For this review, take the finished solid that the model builds, in its own axes (mm). Face numbers are marked on the shaded views. Coordinates: 2 decimals unless noted, no trailing zeros. Loops run counter-clockwise (first coordinate to the right, second up) from the corner with the lowest first, then second, coordinate; pieces in that order, holes last. Notation, with made-up numbers: (66.5, 74) -> (88.5, 74) arc R31 ccw to (88.5, 105) -> close; hole circle Ø2 at (5.5, -3.75). An arc over 180 degrees is marked (long way). Use a Markdown table: item, result.
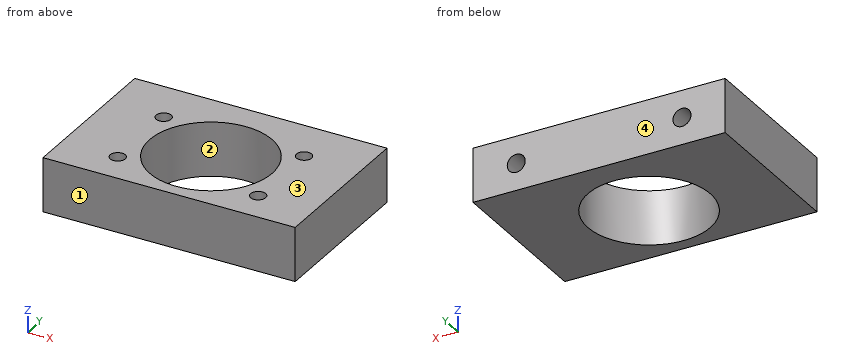
from build123d import *

# Parameters (mm, degrees)
SKETCH_1_W             = 70
SKETCH_1_H             = 45
EXTRUDE_1_DEPTH        = 15
SKETCH_2_R             = 17
CUT_EXTRUDE_1_DEPTH    = 85.557672626
HOLE_WIZARD_M6_1_D     = 5
HOLE_WIZARD_M6_1_DEPTH = 15
HOLE_WIZARD_M6_1_TIP   = 1.502151548
HOLE_WIZARD_M5_1_D     = 4.2
HOLE_WIZARD_M5_1_DEPTH = 12.4
HOLE_WIZARD_M5_1_TIP   = 1.2618073


with BuildPart() as part:
    # 草图1 → 凸台-拉伸1 (new body)
    with BuildSketch(Plane.XY):
        with Locations((35, 22.5)):
            Rectangle(SKETCH_1_W, SKETCH_1_H)
    extrude(amount=EXTRUDE_1_DEPTH)

    # 草图2 → 切除-拉伸1 (cut, through all)
    with BuildSketch(Plane.XY.offset(15)):
        with Locations((35, 20.5)):
            Circle(SKETCH_2_R)
    extrude(amount=-CUT_EXTRUDE_1_DEPTH, mode=Mode.SUBTRACT)

    # M6 螺纹孔1
    with Locations(Plane(origin=(0, 45, 0), x_dir=(-1, 0, 0), z_dir=(0, 1, 0))):
        with Locations((-12, 7.5), (-58, 7.5)):
            Hole(HOLE_WIZARD_M6_1_D / 2, depth=HOLE_WIZARD_M6_1_DEPTH)
            with Locations((0, 0, -(HOLE_WIZARD_M6_1_DEPTH + HOLE_WIZARD_M6_1_TIP / 2))):  # 118° drill point
                Cone(0, HOLE_WIZARD_M6_1_D / 2, HOLE_WIZARD_M6_1_TIP, mode=Mode.SUBTRACT)

    # M5 螺纹孔1
    with Locations(Plane.XY.offset(15)):
        with Locations((54.485571585, 31.75), (15.514428415, 31.75), (54.485571585, 9.25), (15.514428415, 9.25)):
            Hole(HOLE_WIZARD_M5_1_D / 2, depth=HOLE_WIZARD_M5_1_DEPTH)
            with Locations((0, 0, -(HOLE_WIZARD_M5_1_DEPTH + HOLE_WIZARD_M5_1_TIP / 2))):  # 118° drill point
                Cone(0, HOLE_WIZARD_M5_1_D / 2, HOLE_WIZARD_M5_1_TIP, mode=Mode.SUBTRACT)


solid = part.part
(1) Take a section at C-C on z = 11. Write out the cut boundary in (x, y).
Found:
| item | result |
|---|---|
| outline | (0, 0) -> (70, 0) -> (70, 45) -> (0, 45) -> close; hole circle Ø4.2 at (15.51, 9.25); hole circle Ø4.2 at (15.51, 31.75); hole circle Ø34 at (35, 20.5); hole circle Ø4.2 at (54.49, 9.25); hole circle Ø4.2 at (54.49, 31.75) |
(2) Take a section at D-D on y = 27. Write out the cut boundary in (x, z), plus the area to 3 significant figures.
Found:
| item | result |
|---|---|
| outline | (0, 0) -> (19.29, 0) -> (19.29, 15) -> (0, 15) -> close; (50.71, 0) -> (70, 0) -> (70, 15) -> (50.71, 15) -> close |
| area | 579 mm^2 |
(3) For line 1 along Y through (x, z) = (54.5, 4.25); line 2 along X through (y, z) = (32, 2.5); line 3 along Y through (x, z) = (35, 8), list the stretches that pass through material, from the lowest coordinate up.
Found:
| item | result |
|---|---|
| line 1 | y = 0 to 7.15, 11.35 to 29.65, 33.85 to 45 |
| line 2 | x = 0 to 13.6, 17.43 to 22.48, 47.52 to 52.57, 56.4 to 70 |
| line 3 | y = 0 to 3.5, 37.5 to 45 |
(4) Mouldability with a two-part tool opening along Y and no side actions: class the marked faces 1, 2, 3 and 4 as pulls with the +Y half, pulls with the -Y half, needs draft (parallel to the pull), parting line crosses it, or undercut.
Found:
| item | result |
|---|---|
| face 1 | pulls with the -Y half |
| face 2 | undercut |
| face 3 | needs draft |
| face 4 | pulls with the +Y half |
(5) Take a section at B-B on y = 36.5. Write out the cut boundary in (x, z), plus the area to 3 significant figures.
Found:
| item | result |
|---|---|
| outline | (0, 0) -> (29.26, 0) -> (29.26, 15) -> (0, 15) -> close; (40.74, 0) -> (70, 0) -> (70, 15) -> (40.74, 15) -> close; hole circle Ø5 at (12, 7.5); hole circle Ø5 at (58, 7.5) |
| area | 838 mm^2 |
(6) For pin 1 Ø3.5 at (x, y) = (54.49, 31.75) entering from +Z, flat-tipped, find the tip position at first contact; note if it passes through.
Found:
| item | result |
|---|---|
| pin 1 | stops at z = 2.39 |
(7) Take a section at A-A on x = 20. Write out the cut boundary in (y, z).
Found:
| item | result |
|---|---|
| outline | (0, 0) -> (12.5, 0) -> (12.5, 15) -> (0, 15) -> close; (28.5, 0) -> (45, 0) -> (45, 15) -> (28.5, 15) -> close |
